```python
from build123d import *

# Parameters (mm, degrees)
CYLINDER399_R          = 21
CYLINDER399_DEPTH      = 9
BOX330_W               = 26
BOX330_H               = 12
BOX330_DEPTH           = 20
BOX331_W               = 26
BOX331_H               = 15
BOX331_DEPTH           = 25
BOX331_PLACEMENT_ANGLE = 18
CYLINDER407_R          = 4.35
CYLINDER407_DEPTH      = 17
CYLINDER406_R          = 13
CYLINDER406_DEPTH      = 17
CYLINDER403_R          = 1.5
CYLINDER403_DEPTH      = 10
BOX329_W               = 2.5
BOX329_H               = 9
BOX329_DEPTH           = 9
BOX317_W               = 7
BOX317_H               = 2
BOX317_DEPTH           = 17
CYLINDER401_R          = 1.5
CYLINDER401_DEPTH      = 5
CYLINDER397_R          = 1.5
CYLINDER397_DEPTH      = 5
BOX316_W               = 3
BOX316_H               = 2
BOX316_DEPTH           = 9
BOX322_W               = 24
BOX322_H               = 6
BOX322_DEPTH           = 22
CHAMFER_1_SIZE2        = 3
CHAMFER_1_SIZE         = 8
CHAMFER_2_SIZE2        = 3
CHAMFER_2_SIZE         = 8
BOX324_W               = 34
BOX324_H               = 2
BOX324_DEPTH           = 44


with BuildPart() as cone005:
    # Cone004 → Cone004 (revolve)
    with BuildSketch(Plane(origin=(0, 0, 85), x_dir=(1, 0, 0), z_dir=(0, -1, 0))):
        Polygon((0, 0), (21, 0), (5, 41), (0, 41), align=None)
    revolve(axis=Axis((0, 0, 85), (0, 0, 1)))


with BuildPart() as fusion077:
    # Cylinder399 → Cylinder399 (new body)
    with BuildSketch(Plane.XY.offset(76)):
        Circle(CYLINDER399_R)
    extrude(amount=CYLINDER399_DEPTH)

    # Fusion077: union Cone005
    add(cone005.part)


with BuildPart() as cube306:
    # Box330 → Box330 (new body)
    with BuildSketch(Plane(origin=(-13, -14.6, 101), x_dir=(1, 0, 0), z_dir=(0, 0, 1))):
        with Locations((13, 6)):
            Rectangle(BOX330_W, BOX330_H)
    extrude(amount=BOX330_DEPTH)


with BuildPart() as cube307:
    # Box331 → Box331 (new body)
    with BuildSketch(Plane.XY):
        with Locations((13, 7.5)):
            Rectangle(BOX331_W, BOX331_H)
    extrude(amount=BOX331_DEPTH)


with BuildPart() as cube307_1:
    # Box331 placement: moved
    add(cube307.part.moved(Location((-13, -3, 101))).rotate(Axis((-13, -3, 101), (-1, 0, 0)), BOX331_PLACEMENT_ANGLE))


with BuildPart() as cylinder407:
    # Cylinder407 → Cylinder407 (new body)
    with BuildSketch(Plane.XY.offset(103)):
        Circle(CYLINDER407_R)
    extrude(amount=CYLINDER407_DEPTH)


with BuildPart() as antenna_support_carrier:
    # Cylinder406 → Cylinder406 (new body)
    with BuildSketch(Plane.XY.offset(103)):
        Circle(CYLINDER406_R)
    extrude(amount=CYLINDER406_DEPTH)

    # Cut220: cut Cylinder407
    add(cylinder407.part, mode=Mode.SUBTRACT)

    # Cut221: cut Cube307
    add(cube307_1.part, mode=Mode.SUBTRACT)

    # Cut216: cut Cube306
    add(cube306.part, mode=Mode.SUBTRACT)


with BuildPart() as cylinder403:
    # Cylinder403 → Cylinder403 (new body)
    with BuildSketch(Plane(origin=(-20, 1, 72), x_dir=(0, 0, -1), z_dir=(1, 0, 0))):
        Circle(CYLINDER403_R)
    extrude(amount=CYLINDER403_DEPTH)


with BuildPart() as cut223:
    # Box329 → Box329 (new body)
    with BuildSketch(Plane(origin=(-14.5, -4.6, 67), x_dir=(1, 0, 0), z_dir=(0, 0, 1))):
        with Locations((1.25, 4.5)):
            Rectangle(BOX329_W, BOX329_H)
    extrude(amount=BOX329_DEPTH)

    # Cut223: cut Cylinder403
    add(cylinder403.part, mode=Mode.SUBTRACT)


with BuildPart() as cut223_1:
    # Cut223 placement: moved
    add(cut223.part.moved(Location((0, 0, 9))))


with BuildPart() as cube293:
    # Box317 → Box317 (new body)
    with BuildSketch(Plane(origin=(-3.5, -4.6, 103), x_dir=(1, 0, 0), z_dir=(0, 0, 1))):
        with Locations((3.5, 1)):
            Rectangle(BOX317_W, BOX317_H)
    extrude(amount=BOX317_DEPTH)


with BuildPart() as cylinder401:
    # Cylinder401 → Cylinder401 (new body)
    with BuildSketch(Plane(origin=(-8, 0, 100.8), x_dir=(1, 0, 0), z_dir=(0, -1, 0))):
        Circle(CYLINDER401_R)
    extrude(amount=CYLINDER401_DEPTH)


with BuildPart() as screwholes002:
    # Cylinder397 → Cylinder397 (new body)
    with BuildSketch(Plane(origin=(8, 0, 100.8), x_dir=(1, 0, 0), z_dir=(0, -1, 0))):
        Circle(CYLINDER397_R)
    extrude(amount=CYLINDER397_DEPTH)

    # Compound200: union Cylinder401
    add(cylinder401.part)


with BuildPart() as cube292:
    # Box316 → Box316 (new body)
    with BuildSketch(Plane(origin=(-17.5, -4.6, 76), x_dir=(1, 0, 0), z_dir=(0, 0, 1))):
        with Locations((1.5, 1)):
            Rectangle(BOX316_W, BOX316_H)
    extrude(amount=BOX316_DEPTH)


with BuildPart() as cut_outs001:
    # Box322 → Box322 (new body)
    with BuildSketch(Plane(origin=(-12, -4.6, 76), x_dir=(1, 0, 0), z_dir=(0, 0, 1))):
        with Locations((12, 3)):
            Rectangle(BOX322_W, BOX322_H)
    extrude(amount=BOX322_DEPTH)

    # Chamfer 1
    chamfer_1_edges = [cut_outs001.edges().sort_by_distance(p)[0] for p in [
        (12, -1.6, 98),
    ]]
    chamfer_1_side = cut_outs001.faces().sort_by_distance((12, -1.6, 87))[0]
    chamfer(chamfer_1_edges, length=CHAMFER_1_SIZE, length2=CHAMFER_1_SIZE2, reference=chamfer_1_side)

    # Chamfer 2
    chamfer_2_edges = [cut_outs001.edges().sort_by_distance(p)[0] for p in [
        (-12, -1.6, 98),
    ]]
    chamfer_2_side = cut_outs001.faces().sort_by_distance((-12, -1.6, 87))[0]
    chamfer(chamfer_2_edges, length=CHAMFER_2_SIZE, length2=CHAMFER_2_SIZE2, reference=chamfer_2_side)

    # Fusion085: union Cube293, Screwholes002, Cube292
    add(cube293.part)
    add(screwholes002.part)
    add(cube292.part)


with BuildPart() as obj1:
    # Box324 → Box324 (new body)
    with BuildSketch(Plane(origin=(-17, -4.6, 76), x_dir=(1, 0, 0), z_dir=(0, 0, 1))):
        with Locations((17, 1)):
            Rectangle(BOX324_W, BOX324_H)
    extrude(amount=BOX324_DEPTH)

    # Cut225: cut cut-outs001
    add(cut_outs001.part, mode=Mode.SUBTRACT)

    # Fusion086: union Antenna support carrier, Cut223
    add(antenna_support_carrier.part)
    add(cut223_1.part)

    # Common006: intersect Fusion077
    add(fusion077.part, mode=Mode.INTERSECT)


solid = obj1.part
```
The model under review builds one solid part; all positions refer to its coordinate system, in mm. A direction names the side the tool comes from. Coordinates: 2 decimals unless noted, no trailing zeros. Write each loop counter-clockwise with the first axis right and the second up, starting at its lowest first coordinate (ties: lowest second). Pieces come first, ordered by that corner, then holes. Notation, with made-up numbers: (75.25, 79) - (91.25, 79) arc R12 ccw to (91.25, 95) - close; hole circle Ø6 at (21, 71). An arc over 180 degrees is marked (long way). Write item = value, one per line.
(1) Mouldability with a two-part tool opening along X and no side actions: class faces 1 (the face through (-10.479, -3.614, 94.056)), 2 (the face through (-13.27, 1.45, 79.57)), 3 (the face through (-14.5, -1, 80)) as pulls with the +X half, pulls with the -X half, needs draft (parallel to the pull), parting line crosses it, or undercut.
Result sheet:
face_1 = undercut
face_2 = needs draft
face_3 = pulls with the -X half
(2) Consider section C-C, the plane y = 1. State how many separate pieces and enclosed holes the cut face has, then the cut area to 3 significant figures.
Result sheet:
separate_pieces = 4
enclosed_holes = 0
area = 73.3 mm^2
(3) For line 1 (Y direction, x = -13.9, z = 81); line 2 (X direction, y = -3.3, z = 100.8); line 3 (X direction, y = -3.5, z = 100.8), list the stretches that pass through material, from the lowest coordinate up. Write a range as [from, to].
Result sheet:
line_1 = [-4.6, -0.5], [2.5, 4.4]
line_2 = [-14.46, -9.5], [-6.5, 6.5], [9.5, 14.46]
line_3 = [-14.42, -9.5], [-6.5, 6.5], [9.5, 14.42]
(4) For P1, Ø1, axis at x = -16, y = -3.5, coming from the -Z side; P2, Ø2.5, axis at y = -1, z = 80, coming from the +X side; P3, Ø2, axis at y = -3.5, z = 110, coming from the +X side; P4, Ø8, axis at x = -11, z = 112.5, coming from the -Y side, all flat-tipped, find the tip position at first contact; note any pin that passes through.
Result sheet:
P1 = 85
P2 = -12
P3 = 11.19
P4 = -4.6
(5) Machinability: for faces 4 (the face through (12, -4, 83)), 5 (the face through (3.5, -4, 111)), 6 (the face through (-9.885, -2.391, 112.751)), 7 (the face through (-4.24, -0.97, 113.27)), 8 (the face through (-17, -4, 90)), which of the approach directions +Z, -Z, +X, -X, +Y, -Y give a long, thin tool a straight path to every point of the face, cutting with its end or side? Answer none if there is none.
Result sheet:
face_4 = -Z, +Y, -Y
face_5 = +Z, -Y
face_6 = +Z, -X
face_7 = +Z, -Z
face_8 = +Z, -Z, -X, +Y, -Y
(6) Consider section A-A, the plane z = 81. Give the boundary of the cut face in (x, y).
Result sheet:
outline = (-14.5, -4.6) - (-12, -4.6) - (-12, -0.5) - (-14.5, -0.5) - close; (-14.5, 2.5) - (-12, 2.5) - (-12, 4.4) - (-14.5, 4.4) - close; (12, -4.6) - (17, -4.6) - (17, -2.6) - (12, -2.6) - close
(7) Consider section B-B, the plane z = 100.8. Give the boundary of the cut face in (x, y).
Result sheet:
outline = (-14.6, -2.6) arc R14.83 ccw to (-14.1, -4.6) - (-9.5, -4.6) - (-9.5, -2.6) - close; (-6.5, -4.6) - (6.5, -4.6) - (6.5, -2.6) - (-6.5, -2.6) - close; (9.5, -4.6) - (14.1, -4.6) arc R14.83 ccw to (14.6, -2.6) - (9.5, -2.6) - close
